```python
from build123d import *

# Parameters (mm, degrees)
BOSS_EXTRUDE1_DEPTH = 10.16
SKETCH6_W           = 10.16
SKETCH6_H           = 1.27
BOSS_EXTRUDE3_DEPTH = 3.81
SKETCH23_W          = 5.08
SKETCH23_H          = 0.508
BOSS_EXTRUDE4_DEPTH = 2.2225
SKETCH25_W          = 5.08
SKETCH25_H          = 0.508
BOSS_EXTRUDE5_DEPTH = 2.2225
SKETCH26_R          = 1.27
CUT_EXTRUDE1_DEPTH  = 2.2225


with BuildPart() as part:
    # Sketch1 → Boss-Extrude1 (new body)
    with BuildSketch(Plane.XY):
        Polygon((-22.483233333, 11.63955), (-22.483233333, -18.84045), (-18.673233333, -18.84045), (-18.673233333, -20.11045), (-23.753233333, -20.11045), (-23.753233333, 11.63955), align=None)
    extrude(amount=BOSS_EXTRUDE1_DEPTH)

    # Sketch6 → Boss-Extrude3 (add)
    with BuildSketch(Plane(origin=(-22.483233333, 0, 0), x_dir=(0, 0, -1), z_dir=(1, 0, 0))):
        with Locations((-5.08, 2.87655)):
            Rectangle(SKETCH6_W, SKETCH6_H)
    extrude(amount=BOSS_EXTRUDE3_DEPTH)

    # Sketch23 → Boss-Extrude4 (add)
    with BuildSketch(Plane(origin=(-18.673233333, 0, 0), x_dir=(0, 0, -1), z_dir=(1, 0, 0))):
        with Locations((-5.08, 2.87655)):
            Rectangle(SKETCH23_W, SKETCH23_H)
    extrude(amount=BOSS_EXTRUDE4_DEPTH)

    # Sketch25 → Boss-Extrude5 (add)
    with BuildSketch(Plane(origin=(-18.673233333, 0, 0), x_dir=(0, 0, -1), z_dir=(1, 0, 0))):
        with Locations((-5.08, -19.47545)):
            Rectangle(SKETCH25_W, SKETCH25_H)
    extrude(amount=BOSS_EXTRUDE5_DEPTH)

    # Sketch26 → Cut-Extrude1 (cut)
    with BuildSketch(Plane(origin=(-22.483233333, 0, 0), x_dir=(0, 0, -1), z_dir=(1, 0, 0))):
        with Locations((-5.111682079, 8.84555)):
            Circle(SKETCH26_R)
    extrude(amount=-CUT_EXTRUDE1_DEPTH, mode=Mode.SUBTRACT)


solid = part.part
```
For this review, take the finished solid that the model builds, in its own axes (mm). A direction names the side the tool comes from. Give positions to 0.01 mm unless a question says otherwise; leave off trailing zeros. Write each loop counter-clockwise with the first axis right and the second up, starting at its lowest first coordinate (ties: lowest second). Pieces come first, ordered by that corner, then holes. Notation, with made-up numbers: M 31.25,-23.75 L 51.25,-23.75 A19 ccw 51.25,-1.75 Z; hole C -24,52.25 d6. An arc over 180 degrees is marked long. One line per item, written item: value.
1) Take a section at C-C, the plane z = 8.5. Write out the cut boundary in (x, y), then the cut area to 3 significant figures.
Results are:
outline: M -23.75,-20.11 L -18.67,-20.11 L -18.67,-18.84 L -22.48,-18.84 L -22.48,2.24 L -18.67,2.24 L -18.67,3.51 L -22.48,3.51 L -22.48,11.64 L -23.75,11.64 Z
area: 50.0 mm²
2) Take a section at D-D, the plane z = 4.25. Write out the cut boundary in (x, y), then the cut area to 3 significant figures.
Results are:
outline: M -23.75,-20.11 L -18.67,-20.11 L -18.67,-19.73 L -16.45,-19.73 L -16.45,-19.22 L -18.67,-19.22 L -18.67,-18.84 L -22.48,-18.84 L -22.48,2.24 L -18.67,2.24 L -18.67,2.62 L -16.45,2.62 L -16.45,3.13 L -18.67,3.13 L -18.67,3.51 L -22.48,3.51 L -22.48,7.91 L -23.75,7.91 Z; M -23.75,9.78 L -22.48,9.78 L -22.48,11.64 L -23.75,11.64 Z
area: 49.9 mm²
3) For faces 5 (the flat face through (-23, 11.64, 5)), 6 (the flat face through (-18, 2.623, 5)), 7 (the flat face through (-18, -19.729, 5)), 8 (the flat face through (-21, -20.11, 5)), 9 (the flat face through (-18, 3.131, 5)), list the 3-axis set-ups (+Z, -Z, +X, -X, +Y, -Y) from which the entire face can be reached by the end or side of a thin tool; tool diameter is ignored.
Results are:
face 5: +Z, -Z, +X, -X, +Y
face 6: +Z, -Z, +X
face 7: +Z, -Z, +X, -Y
face 8: +Z, -Z, +X, -X, -Y
face 9: +Z, -Z, +X, +Y
4) For line 1 (Y direction, x = -21, z = 5.75); line 2 (Y direction, x = -18.25, z = 6.5); line 3 (X direction, y = -4, z = 7.25), list the stretches that pass through material, from the lowest coordinate up. Write a range as from..to.
Results are:
line 1: y = -20.11..-18.84, 2.24..3.51
line 2: y = -19.73..-19.22, 2.62..3.13
line 3: x = -23.75..-22.48
5) The part is to be moulded in two halves that separate along Z. For faces 1 (the flat face through (-23, -5, 10.16)), 2 (the flat face through (-23, -5, 0)), 3 (the cylindrical face through (-23.109, 7.719, 4.526)), 4 (the flat face through (-22.483, -8, 5)), say which applies: +Z half, -Z half, draft (parallel to the pull), parting line (faces both ways), or undercut.
Results are:
face 1: +Z half
face 2: -Z half
face 3: undercut
face 4: draft
6) Take a section at A-A, the plane x = -17.25. Write out the cut boundary in (y, z).
Results are:
outline: M -19.73,2.54 L -19.22,2.54 L -19.22,7.62 L -19.73,7.62 Z; M 2.62,2.54 L 3.13,2.54 L 3.13,7.62 L 2.62,7.62 Z
7) Take a section at B-B, the plane y = 8.5. Write out the cut boundary in (x, z).
Results are:
outline: M -23.75,0 L -22.48,0 L -22.48,3.89 L -23.75,3.89 Z; M -23.75,6.33 L -22.48,6.33 L -22.48,10.16 L -23.75,10.16 Z
8) For P1, Ø0.7, axis at x = -18, z = 4.5, coming from the -Y side; P2, Ø2.5, axis at x = -18, z = 5, coming from the +Y side; P3, Ø0.6, axis at x = -18, y = -19.5, coming from the +Z side; P4, Ø6, axis at y = 1, z = 8, coming from the +X side, all flat-tipped, find the tip position at first contact; note any pin that passes through.
Results are:
P1: stops at y = -19.73
P2: stops at y = 3.51
P3: stops at z = 7.62
P4: stops at x = -16.45
